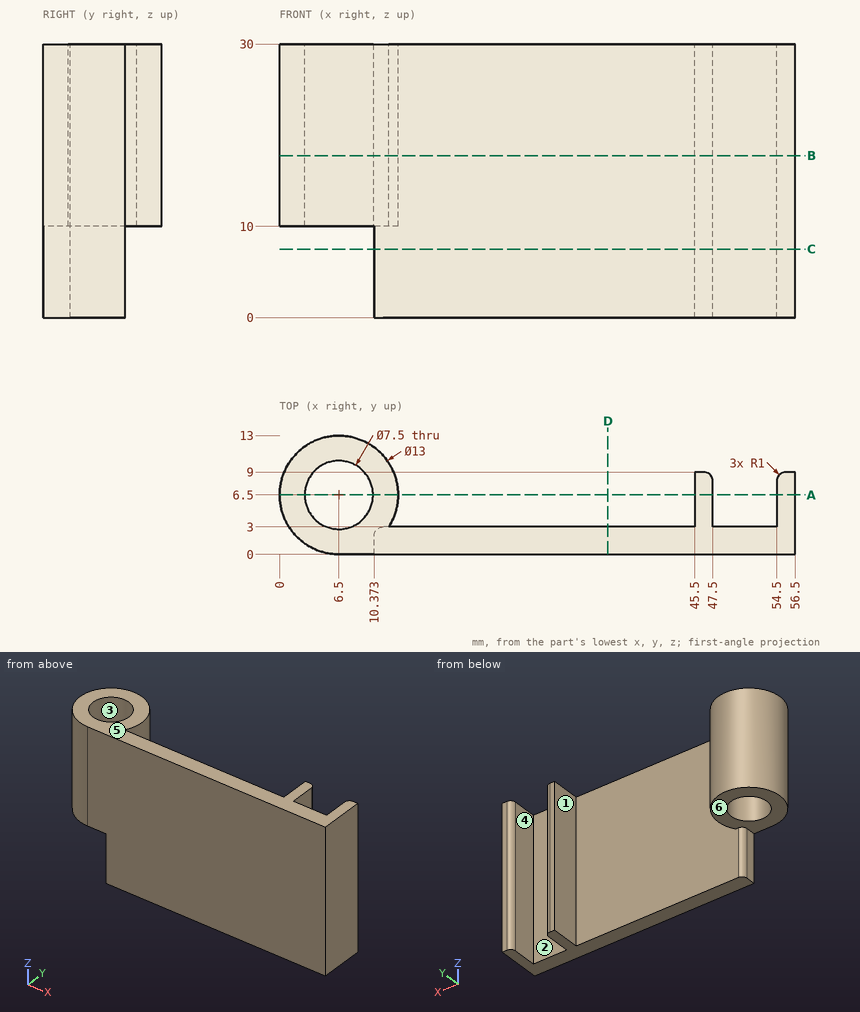
The drawing under review shows one solid part. Ordinate dimensions are in mm from its lowest x, y, z. A direction names the side the tool comes from. Coordinates: 2 decimals unless noted, no trailing zeros. Order: outer loops, then holes, each group sorted by start corner. A loop starts at its lowest first (then second) coordinate and runs counter-clockwise, first axis right, second up. Notation, with made-up numbers: (-17, 13) -> (34, 13) arc R19 ccw to (34, 30) -> close; hole circle Ø9 at (18.5, 63). An arc over 180 degrees is marked (long way). One line per item, written item: value.
1) We need section D-D, the plane x = 36. Give the boundary of the cut face in (y, z), then the cut area to 3 significant figures.
Output values:
outline: (0, 0) -> (3, 0) -> (3, 30) -> (0, 30) -> close
area: 90.0 mm2
2) To check wall thickness, follow probe 1 along Y at (x, z) = (6.5, 21.75); probe 2 along X at (y, z) = (4, 8.5); probe 3 along Z at (x, y) = (12, 8.75). State the ranges of each line that lie inside material, in increasing order. Write a range as [from, to].
Output values:
probe 1: y = [0, 2.75], [10.25, 13]
probe 2: x = [45.5, 47.5], [54.5, 56.5]
probe 3: z = [10, 30]
3) We need section A-A, the plane y = 6.5. Give the boundary of the cut face in (x, z), then the cut area to 3 significant figures.
Output values:
outline: (0, 10) -> (2.75, 10) -> (2.75, 30) -> (0, 30) -> close; (10.25, 10) -> (13, 10) -> (13, 30) -> (10.25, 30) -> close; (45.5, 0) -> (47.5, 0) -> (47.5, 30) -> (45.5, 30) -> close; (54.5, 0) -> (56.5, 0) -> (56.5, 30) -> (54.5, 30) -> close
area: 230 mm2
4) Clearance check with flat-ended pins moving along their axes: P1, Ø12, axis at x = 15, z = 19.5, coming from the +Y side; P2, Ø3.5, axis at x = 49.5, z = 15.5, coming from the +Y side; P3, Ø6.5, axis at x = 5.5, y = 5.5, coming from the -Z side. State where each tip first meets the part, or that it passes through.
Output values:
P1: stops at y = 12.5
P2: stops at y = 3
P3: stops at z = 10
5) Draft analysis for pull direction Y (two halves, no side actions). For the marked faces 1, 2 and 3, state which applies: +Y half, -Y half, draft (parallel to the pull), parting line (faces both ways), or undercut.
Output values:
face 1: draft
face 2: +Y half
face 3: undercut
6) We need section B-B, the plane z = 17.75. Give the boundary of the cut face in (x, y).
Output values:
outline: (6.5, 0) -> (56.5, 0) -> (56.5, 9) -> (55.5, 9) arc R1 ccw to (54.5, 8) -> (54.5, 3) -> (47.5, 3) -> (47.5, 8) arc R1 ccw to (46.5, 9) -> (45.5, 9) -> (45.5, 3) -> (11.98, 3) arc R6.5 ccw (long way) to start; hole circle Ø7.5 at (6.5, 6.5)
7) Machinability: for the marked faces 4, 5 and 6, which of the approach directions +Z, -Z, +X, -X, +Y, -Y give a long, thin tool a straight path to every point of the face, cutting with its end or side? Answer none if there is none.
Output values:
face 4: +Z, -Z, +Y
face 5: +Z, +X, -X, +Y, -Y
face 6: -Z, -X, +Y
8) We need section C-C, the plane z = 7.5. Give the boundary of the cut face in (x, y), then the cut area to 3 significant figures.
Output values:
outline: (10.37, 0) -> (56.5, 0) -> (56.5, 9) -> (55.5, 9) arc R1 ccw to (54.5, 8) -> (54.5, 3) -> (47.5, 3) -> (47.5, 8) arc R1 ccw to (46.5, 9) -> (45.5, 9) -> (45.5, 3) -> (11.37, 3) arc R1 ccw to (10.37, 2) -> close
area: 162 mm2
